Design review of the part built by this model. Coordinates are the model's own, in mm. Round coordinates to 2 decimals unless told otherwise and drop trailing zeros. Loops run counter-clockwise (first coordinate to the right, second up) from the corner with the lowest first, then second, coordinate; pieces in that order, holes last. Notation, with made-up numbers: (33, 46) - (48, 46) arc R26 ccw to (48, 65) - close; hole circle Ø1 at (12.5, 23.25). An arc over 180 degrees is marked (long way). Answer as CSV lines item,"result". Start each with the question number.
(1) Consider section B-B (x = -16). Give the boundary of the cut face in (y, z).
(2) Wall thickness on L1, parallel to Y at x = -134.65, z = 2.45; L2, parallel to X at y = -29.5, z = 2.95; L3, parallel to X at y = -16.5, z = 0.85: over which ranges is each line inside the solid? List them lowest first.
(3) Consider section A-A (z = 0.75). Count the separate pieces of the cut face and the enclosed holes in it, and give its area (3 significant figures).
(4) For P1, Ø2, axis at x = -64.5, z = 2.5, coming from the +Y side; P2, Ø1.9, axis at x = -134.65, y = -37.5, coming from the +Z side; P3, Ø2, axis at x = 84, y = -32, coming from the +Z side, all flat-tipped, find the tip position at first contact; note any pin that passes through.
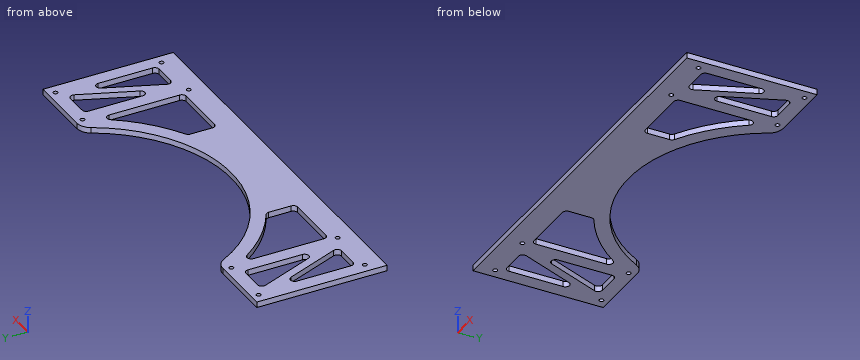
from build123d import *

# Parameters (mm, degrees)
BOSS_EXTRUDE1_DEPTH = 4
SKETCH2_R           = 1.55
CUT_EXTRUDE1_DEPTH  = 10
FILLET1_R           = 10
SKETCH3_W           = 283.3
SKETCH3_H           = 4
BOSS_EXTRUDE2_DEPTH = 6.958779143


with BuildPart() as part:
    # Sketch1 → Boss-Extrude1 (new body)
    with BuildSketch(Plane.XY):
        with BuildLine():
            Line((-141.65, 42.5), (-141.65, -42.5))
            Line((-141.65, -42.5), (141.65, -42.5))
            Line((141.65, -42.5), (141.65, 42.5))
            Line((141.65, 42.5), (90.519334951, 42.5))
            ThreePointArc((90.519334951, 42.5), (0, -15), (-90.519334951, 42.5))
            Line((-90.519334951, 42.5), (-141.65, 42.5))
        make_face()
    extrude(amount=BOSS_EXTRUDE1_DEPTH)

    # Sketch2 → Cut-Extrude1 (cut)
    with BuildSketch(Plane.XY.offset(4)):
        with BuildLine():
            Line((-125.864569927, 9.958677608), (-110.526767696, -28.385827971))
            ThreePointArc((-110.526767696, -28.385827971), (-110.827996077, -31.181886428), (-113.312197769, -32.5))
            Line((-113.312197769, -32.5), (-128.65, -32.5))
            ThreePointArc((-128.65, -32.5), (-130.771320344, -31.621320344), (-131.65, -29.5))
            Line((-131.65, -29.5), (-131.65, 8.844505579))
            ThreePointArc((-131.65, 8.844505579), (-129.217322563, 11.790374739), (-125.864569927, 9.958677608))
        make_face()
        with BuildLine():
            ThreePointArc((-126.773232304, 28.385827971), (-126.472003923, 31.181886428), (-123.987802231, 32.5))
            Line((-123.987802231, 32.5), (-108.65, 32.5))
            ThreePointArc((-108.65, 32.5), (-106.528679656, 31.621320344), (-105.65, 29.5))
            Line((-105.65, 29.5), (-105.65, -8.844505579))
            ThreePointArc((-105.65, -8.844505579), (-108.082677437, -11.790374739), (-111.435430073, -9.958677608))
            Line((-111.435430073, -9.958677608), (-126.773232304, 28.385827971))
        make_face()
        with BuildLine():
            ThreePointArc((-95.65, 20.308597944), (-93.550221212, 23.170345971), (-90.190265487, 22.026068795))
            ThreePointArc((-90.190265487, 22.026068795), (-73.741634921, 3.377875064), (-53.524791107, -11.0994107))
            ThreePointArc((-53.524791107, -11.0994107), (-52.39812226, -12.200320346), (-51.984558137, -13.72030372))
            Line((-51.984558137, -13.72030372), (-51.984558137, -29.5))
            ThreePointArc((-51.984558137, -29.5), (-52.863237794, -31.621320344), (-54.984558137, -32.5))
            Line((-54.984558137, -32.5), (-92.65, -32.5))
            ThreePointArc((-92.65, -32.5), (-94.771320344, -31.621320344), (-95.65, -29.5))
            Line((-95.65, -29.5), (-95.65, 20.308597944))
        make_face()
        with BuildLine():
            ThreePointArc((95.65, 20.308597944), (93.550221212, 23.170345971), (90.190265487, 22.026068795))
            ThreePointArc((90.190265487, 22.026068795), (73.741634921, 3.377875064), (53.524791107, -11.0994107))
            ThreePointArc((53.524791107, -11.0994107), (52.39812226, -12.200320346), (51.984558137, -13.72030372))
            Line((51.984558137, -13.72030372), (51.984558137, -29.5))
            ThreePointArc((51.984558137, -29.5), (52.863237794, -31.621320344), (54.984558137, -32.5))
            Line((54.984558137, -32.5), (92.65, -32.5))
            ThreePointArc((92.65, -32.5), (94.771320344, -31.621320344), (95.65, -29.5))
            Line((95.65, -29.5), (95.65, 20.308597944))
        make_face()
        with BuildLine():
            ThreePointArc((111.435430073, -9.958677608), (108.082677437, -11.790374739), (105.65, -8.844505579))
            Line((105.65, -8.844505579), (105.65, 29.5))
            ThreePointArc((105.65, 29.5), (106.528679656, 31.621320344), (108.65, 32.5))
            Line((108.65, 32.5), (123.987802231, 32.5))
            ThreePointArc((123.987802231, 32.5), (126.472003923, 31.181886428), (126.773232304, 28.385827971))
            Line((126.773232304, 28.385827971), (111.435430073, -9.958677608))
        make_face()
        with BuildLine():
            Line((128.65, -32.5), (113.312197769, -32.5))
            ThreePointArc((113.312197769, -32.5), (110.827996077, -31.181886428), (110.526767696, -28.385827971))
            Line((110.526767696, -28.385827971), (125.864569927, 9.958677608))
            ThreePointArc((125.864569927, 9.958677608), (129.217322563, 11.790374739), (131.65, 8.844505579))
            Line((131.65, 8.844505579), (131.65, -29.5))
            ThreePointArc((131.65, -29.5), (130.771320344, -31.621320344), (128.65, -32.5))
        make_face()
        with Locations((-134.65, 37.5)):
            Circle(SKETCH2_R)
        with Locations((-98.65, 37.5)):
            Circle(SKETCH2_R)
        with Locations((-98.65, -37.5)):
            Circle(SKETCH2_R)
        with Locations((-134.65, -37.5)):
            Circle(SKETCH2_R)
        with Locations((98.65, -37.5)):
            Circle(SKETCH2_R)
        with Locations((134.65, -37.5)):
            Circle(SKETCH2_R)
        with Locations((98.65, 37.5)):
            Circle(SKETCH2_R)
        with Locations((134.65, 37.5)):
            Circle(SKETCH2_R)
    extrude(amount=-CUT_EXTRUDE1_DEPTH, mode=Mode.SUBTRACT)

    # Fillet1
    fillet1_edges = [part.edges().sort_by_distance(p)[0] for p in [
        (90.519334951, 42.5, 2),
        (-90.519334951, 42.5, 2),
    ]]
    fillet(fillet1_edges, radius=FILLET1_R)

    # Sketch3 → Boss-Extrude2 (add)
    with BuildSketch(Plane.XZ.offset(42.5)):
        with Locations((0, 2)):
            Rectangle(SKETCH3_W, SKETCH3_H)
    extrude(amount=BOSS_EXTRUDE2_DEPTH)


solid = part.part
Determined:
1,outline,"(-49.46, 0) - (-13.71, 0) - (-13.71, 4) - (-49.46, 4) - close"
2,L1,"y = -49.46 to -39.05, -35.95 to 35.95, 39.05 to 42.5"
2,L2,"x = -141.65 to -131.65, -110.31 to -95.65, -51.98 to 51.98, 95.65 to 110.31, 131.65 to 141.65"
2,L3,"x = -141.65 to -131.65, -115.28 to -95.65, -51.98 to 51.98, 95.65 to 115.28, 131.65 to 141.65"
3,separate pieces,"1"
3,enclosed holes,"14"
3,area,"12,800 mm^2"
4,P1,"stops at y = 9.44"
4,P2,"passes through"
4,P3,"stops at z = 4"
